Design review of the part shown in the three views and the two pictorial views. Dimensions are in mm from the part's minimum x, y and z. A direction names the side the tool comes from. Coordinates: 2 decimals unless noted, no trailing zeros. Order: outer loops, then holes, each group sorted by start corner. A loop starts at its lowest first (then second) coordinate and runs counter-clockwise, first axis right, second up. Notation, with made-up numbers: (-26, -7) - (-3, -7) arc R17 ccw to (-3, 6) - close; hole circle Ø4 at (-12.75, -24.5). An arc over 180 degrees is marked (long way). One line per item, written item: value. Start each with the question number.
(1) Mouldability with a two-part tool opening along Z and no side actions: class the marked faces 1, 2 and 3 as released by +Z, released by -Z, zero draft, split by the parting line, or undercut.
(2) Clearance check with flat-ended pins moving along their axes: pin 1 (4 mm diameter, centred on x = 5, z = 2, fed in from -Y); pin 2 (2.5 mm diameter, centred on y = 2.75, z = 4.5, fed in from +X); pin 3 (1.4 mm diameter, centred on x = 19, y = 3.5, fed in from -Z); pin 4 (3 mm diameter, centred on x = 3, y = 6, fed in from +Z). State where each tip first meets the part, or that it passes through.
(3) For the marked faces 4 and 5, list the 3-axis set-ups (+Z, -Z, +X, -X, +Y, -Y) from which the entire face can be reached by the end or side of a thin tool; tool diameter is ignored.
(4) Consider section A-A on z = 4.5. Write out the cut boundary in (x, y).
(5) To check wall thickness, follow line 1 along Y through (x, z) = (4.5, 4.5); line 2 along Y through (x, z) = (17.75, 4.5); line 3 along Z through (x, y) = (13.25, 7.75). State the ranges of each line that lie inside material, in increasing order.
(6) Consider section D-D on y = 7.75. Write out the cut boundary in (x, z).
(7) Consider section B-B on y = 9.5. Write out the cut boundary in (x, z) (1 decimal).
(8) Consider section C-C on x = 5. Count the separate pieces of the cut face and the enclosed holes in it.
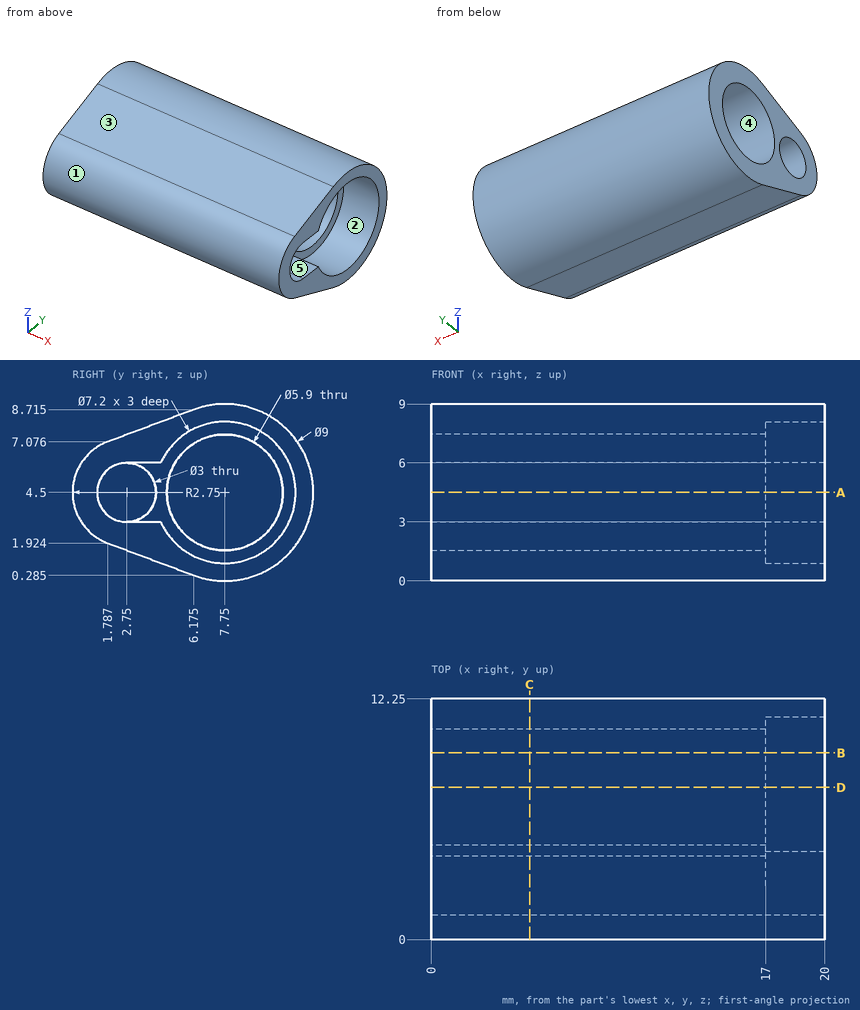
Geometry check:
1. face 1: split by the parting line
1. face 2: undercut
1. face 3: released by +Z
2. pin 1: stops at y = 0.05
2. pin 2: passes through
2. pin 3: stops at z = 1.02
2. pin 4: stops at z = 8.99
3. face 4: +X, -X
3. face 5: +X
4. outline: (0, 0) - (20, 0) - (20, 1.25) - (0, 1.25) - close; (0, 4.25) - (17, 4.25) - (17, 4.8) - (0, 4.8) - close; (0, 10.7) - (17, 10.7) - (17, 11.35) - (20, 11.35) - (20, 12.25) - (0, 12.25) - close
5. line 1: y = 0 to 1.25, 4.25 to 4.8, 10.7 to 12.25
5. line 2: y = 0 to 1.25, 11.35 to 12.25
5. line 3: z = 0 to 1.55, 7.45 to 9
6. outline: (0, 0) - (20, 0) - (20, 0.9) - (17, 0.9) - (17, 1.55) - (0, 1.55) - close; (0, 7.45) - (17, 7.45) - (17, 8.1) - (20, 8.1) - (20, 9) - (0, 9) - close
7. outline: (0, 0.4) - (20, 0.4) - (20, 1.4) - (17, 1.4) - (17, 2.1) - (0, 2.1) - close; (0, 6.9) - (17, 6.9) - (17, 7.6) - (20, 7.6) - (20, 8.6) - (0, 8.6) - close
8. separate pieces: 1
8. enclosed holes: 2
